from build123d import *

# Parameters (mm, degrees)
SKIZZE1_W                       = 200
SKIZZE1_H                       = 150
AUFSATZ_LINEAR_AUSTRAGEN1_DEPTH = 1
SCHNITT_LINEAR_AUSTRAGEN5_DEPTH = 2
LINEARES_MUSTER2_COUNT          = 5
LINEARES_MUSTER2_PITCH          = 28
LINEARES_MUSTER2_COUNT_DIR2     = 3
LINEARES_MUSTER2_PITCH_DIR2     = 26
SCHNITT_LINEAR_AUSTRAGEN6_DEPTH = 2
LINEARES_MUSTER3_COUNT          = 5
LINEARES_MUSTER3_PITCH          = 28
LINEARES_MUSTER3_COUNT_DIR2     = 3
LINEARES_MUSTER3_PITCH_DIR2     = 26
SKIZZE9_R                       = 5
SCHNITT_LINEAR_AUSTRAGEN7_DEPTH = 2


with BuildPart() as part:
    # Skizze1 → Aufsatz-Linear austragen1 (new body)
    with BuildSketch(Plane.XY):
        with Locations((100, 75)):
            Rectangle(SKIZZE1_W, SKIZZE1_H)
    extrude(amount=AUFSATZ_LINEAR_AUSTRAGEN1_DEPTH)

    # Langlochmuster → Schnitt-Linear austragen5 (cut, through all)
    with BuildSketch(Plane.XY.offset(1)):
        with BuildLine():
            Line((28.425192668, 34.450971961), (43.425192668, 34.450971961))
            ThreePointArc((43.425192668, 34.450971961), (48.425192668, 29.450971961), (43.425192668, 24.450971961))
            Line((43.425192668, 24.450971961), (28.425192668, 24.450971961))
            ThreePointArc((28.425192668, 24.450971961), (23.425192668, 29.450971961), (28.425192668, 34.450971961))
        make_face()
    schnitt_linear_austragen5 = extrude(amount=-SCHNITT_LINEAR_AUSTRAGEN5_DEPTH, mode=Mode.SUBTRACT)

    # Lineares Muster2: Schnitt-Linear austragen5 5 × 3, 2 skipped
    with Locations(*[(i * LINEARES_MUSTER2_PITCH, j * LINEARES_MUSTER2_PITCH_DIR2, 0) for i in range(LINEARES_MUSTER2_COUNT) for j in range(LINEARES_MUSTER2_COUNT_DIR2) if (i, j) not in ((0, 0), (0, 2), (1, 2))]):
        add(schnitt_linear_austragen5, mode=Mode.SUBTRACT)

    # Skizze8_3 → Schnitt-Linear austragen6 (cut, through all)
    with BuildSketch(Plane.XY.offset(1)):
        with BuildLine():
            Line((42.425192668, 47.450971961), (57.425192668, 47.450971961))
            ThreePointArc((57.425192668, 47.450971961), (62.425192668, 42.450971961), (57.425192668, 37.450971961))
            Line((57.425192668, 37.450971961), (42.425192668, 37.450971961))
            ThreePointArc((42.425192668, 37.450971961), (37.425192668, 42.450971961), (42.425192668, 47.450971961))
        make_face()
    schnitt_linear_austragen6 = extrude(amount=-SCHNITT_LINEAR_AUSTRAGEN6_DEPTH, mode=Mode.SUBTRACT)

    # Lineares Muster3: Schnitt-Linear austragen6 5 × 3, 4 skipped
    with Locations(*[(i * LINEARES_MUSTER3_PITCH, j * LINEARES_MUSTER3_PITCH_DIR2, 0) for i in range(LINEARES_MUSTER3_COUNT) for j in range(LINEARES_MUSTER3_COUNT_DIR2) if (i, j) not in ((0, 0), (0, 2), (1, 2), (2, 2), (4, 2))]):
        add(schnitt_linear_austragen6, mode=Mode.SUBTRACT)

    # Skizze9 → Schnitt-Linear austragen7 (cut, through all)
    with BuildSketch(Plane.XY.offset(1)):
        with Locations((28.425192668, 42.450971961)):
            Circle(SKIZZE9_R)
        with Locations((112.425192668, 94.450971961)):
            Circle(SKIZZE9_R)
        with Locations((169.425192668, 55.450971961)):
            Circle(SKIZZE9_R)
        with Locations((169.425192668, 29.450971961)):
            Circle(SKIZZE9_R)
    extrude(amount=-SCHNITT_LINEAR_AUSTRAGEN7_DEPTH, mode=Mode.SUBTRACT)


solid = part.part
Part model, mm, in its own coordinate system. Coordinates: 2 decimals unless noted, no trailing zeros. Order: outer loops, then holes, each group sorted by start corner. A loop starts at its lowest first (then second) coordinate and runs counter-clockwise, first axis right, second up.
(1) Pin check, flat tips, straight feed: pin 1 Ø0.5 at (x, z) = (49.5, 0.5) entering from -Y; pin 2 Ø6 at (x, y) = (169.43, 29.45) entering from +Z. Stop position of each tip, or through.
Check sheet entries:
pin 1: stops at y = 0
pin 2: passes through
(2) Probe L1, parallel to Y at x = 79, z = 0.55; L2, parallel to Y at x = 146.5, z = 0.8; L3, parallel to Y at x = 86, z = 0.3. List the from-to ranges inside material, lowest first.
Check sheet entries:
L1: y = 0 to 37.45, 47.45 to 63.45, 73.45 to 150
L2: y = 0 to 24.45, 34.45 to 50.45, 60.45 to 76.45, 86.45 to 150
L3: y = 0 to 24.45, 34.45 to 37.48, 47.42 to 50.45, 60.45 to 63.48, 73.42 to 76.45, 86.45 to 150
(3) Slice it at C-C, the plane z = 0.2. State how many separate pieces and enclosed holes the cut face has, and give its area (3 significant figures).
Check sheet entries:
separate pieces: 1
enclosed holes: 28
area: 24,200 mm2
(4) Pull direction X, two halves, no side cores. Call faces 1 (the face through (171.7, 51, 0.5)), 2 (the face through (99, 76, 0)): pulls with the +X half, pulls with the -X half, needs draft (parallel to the pull), parting line crosses it, or undercut.
Check sheet entries:
face 1: undercut
face 2: needs draft
(5) Slice it at A-A, the plane x = 102. Write the cut outline in (y, z), and give its area (3 significant figures).
Check sheet entries:
outline: (0, 0) - (25.16, 0) - (25.16, 1) - (0, 1) - close; (33.74, 0) - (37.45, 0) - (37.45, 1) - (33.74, 1) - close; (47.45, 0) - (51.16, 0) - (51.16, 1) - (47.45, 1) - close; (59.74, 0) - (63.45, 0) - (63.45, 1) - (59.74, 1) - close; (73.45, 0) - (77.16, 0) - (77.16, 1) - (73.45, 1) - close; (85.74, 0) - (150, 0) - (150, 1) - (85.74, 1) - close
area: 104 mm2
(6) Slice it at B-B, the plane x = 167. Write the cut outline in (y, z).
Check sheet entries:
outline: (0, 0) - (25.08, 0) - (25.08, 1) - (0, 1) - close; (33.82, 0) - (37.45, 0) - (37.45, 1) - (33.82, 1) - close; (47.45, 0) - (51.08, 0) - (51.08, 1) - (47.45, 1) - close; (59.82, 0) - (63.45, 0) - (63.45, 1) - (59.82, 1) - close; (73.45, 0) - (150, 0) - (150, 1) - (73.45, 1) - close
